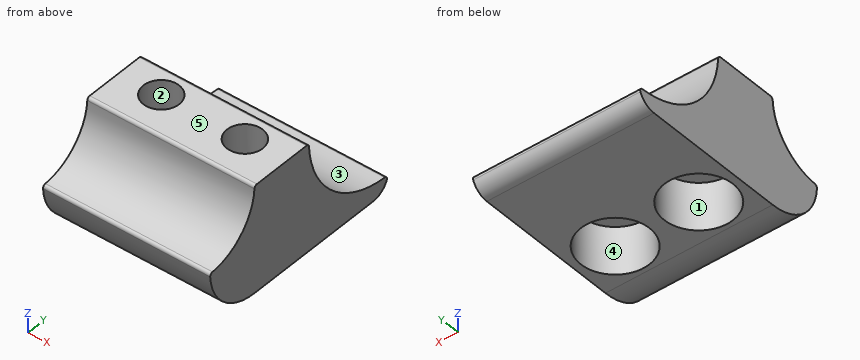
Autodesk Inventor part; units mm, degrees
ref_plane "YZ Plane" through (0, 0, 0) normal (1, 0, 0) x (0, 1, 0)
ref_plane "XZ Plane" through (0, 0, 0) normal (0, 1, 0) x (-1, 0, 0)
ref_plane "XY Plane" through (0, 0, 0) normal (0, 0, 1) x (1, 0, 0)
sketch "Szkic1" plane through (0, 0, 0) normal (0, 0, 1) x (1, 0, 0)
  line L0 (-14, 18) -> (14, 18)
  line L1 (14, 18) -> (14, -18)
  line L2 (14, -18) -> (-14, -18)
  line L3 (-14, -18) -> (-14, 18)
  line L4 (-14, 18) -> (14, -18) construction
  line L5 (14, 18) -> (-14, -18) construction
  point P0 (0, 0)
  dimension "d0" = 28
  dimension "d1" = 36
extrude "Wyciągnięcie proste1" add sketch "Szkic1" along normal mid plane 18
sketch "Szkic3" plane through (0, 0, 0) normal (1, 0, 0) x (0, 1, 0)
  line L0 (-18, 9) -> (-18, -9) construction
  line L1 (-18, 9) -> (18, 9) construction
  line L2 (18, 9) -> (18, -9) construction
  circle A0 centre (-18, 9) radius 9
  circle A1 centre (18, 9.5) radius 16
  point P0 (0, 0)
  dimension "d4" = 18
  dimension "d6" = 32
  dimension "d7" = 0.5
extrude "Wyciągnięcie proste2" cut sketch "Szkic3" along normal mid plane 28
fillet "Zaokrąglenie1" radius 3 1 edges at (0, 18, -9)
fillet "Zaokrąglenie2" radius 9 1 edges at (0, -18, -9)
fillet "Zaokrąglenie3" radius 0.5 5 edges at (0, -9, 9) (0, 2.0078, 9) (0, -18, -0.0001) (0, -18, 0) (0, 18, -6.5)
sketch "Szkic4" plane through (0, 0, -9) normal (0, 0, -1) x (-1, 0, 0)
  line L0 (14, -9) -> (-14, -9)
  line L1 (14, -9) -> (14, 15.042)
  line L2 (-14, 15.042) -> (14, 15.042)
  line L3 (-14, 15.042) -> (-14, -9)
  line L4 (-14, 2.0294) -> (14, 2.0294)
  line L5 (14, -9.0125) -> (-14, -9.0125)
  line L6 (0, 0) -> (0, 3.9534) construction
  point P0 (-7, -2.4906)
  point P1 (7, -2.4906)
  point P2 (-12.5, 2.0294)
  point P3 (12.5, 2.0294)
  point P4 (12.5, -7.0104)
  point P5 (-12.5, -7.0104)
  dimension "d14" = 4.52
  dimension "d15" = 14
hole "Otwór1" at (7, -2.4906, -9) at (-7, -2.4906, -9) direction (0, 0, 1) diameter 6 end through all counterbore diameter 11.5 counterbore depth 8
properties part number "Zawias" material "Stal nierdzewna"
Design review of the part built by this model. Coordinates are the model's own, in mm. Face numbers are marked on the shaded views. A direction names the side the tool comes from. Round coordinates to 2 decimals unless told otherwise and drop trailing zeros. Write each loop counter-clockwise with the first axis right and the second up, starting at its lowest first coordinate (ties: lowest second). Pieces come first, ordered by that corner, then holes. Notation, with made-up numbers: M -5,71.25 L 51,71.25 A36 ccw 51,105.25 Z; hole C 60.5,84.25 d11. An arc over 180 degrees is marked long. One line per item, written item: value. Start each with the question number.
1. Draft analysis for pull direction Y (two halves, no side actions). For the marked faces 3, 4 and 5, state which applies: pulls with the +Y half, pulls with the -Y half, needs draft (parallel to the pull), parting line crosses it, or undercut.
2. Take a section at A-A on z = 1.5. State the section outline as (x, y) points.
3. Clearance check with flat-ended pins moving along their axes: P1, Ø9, axis at x = 6.5, y = -2.5, coming from the -Z side; P2, Ø4, axis at x = -6.5, y = 14, coming from the +Z side; P3, Ø2, axis at x = 7, z = 2, coming from the +Y side. State where each tip first meets the part, or that it passes through.
4. For the marked faces 1 and 2, list the 3-axis set-ups (+Z, -Z, +X, -X, +Y, -Y) from which the entire face can be reached by the end or side of a thin tool; tool diameter is ignored.
5. To check wall thickness, follow probe 1 along X at (y, z) = (-3, 4); probe 2 along X at (y, z) = (-7.5, -4.75); probe 3 along Y at (x, z) = (-7, -4). State the ranges of each line that lie inside material, in increasing order. Write a range as from..to.
6. Take a section at C-C on y = -15. State the section outline as (x, z) points, then the cut area to 3 significant figures.
7. Take a section at B-B on z = -3. State the section outline as (x, y) points, then the cut area to 3 significant figures.
8. Take a section at D-D on y = 7. State the section outline as (x, z) points.
Computed:
1. face 3: pulls with the +Y half
1. face 4: undercut
1. face 5: needs draft
2. outline: M -14,-13.03 L 14,-13.03 L 14,4.14 L -14,4.14 Z; hole C -7,-2.49 d6; hole C 7,-2.49 d6
3. P1: stops at z = -1
3. P2: stops at z = -5.33
3. P3: stops at y = 4.44
4. face 1: -Z
4. face 2: +Z, -Z
5. probe 1: x = -14..-9.96, -4.04..4.04, 9.96..14
5. probe 2: x = -14..-9.82, -4.18..4.18, 9.82..14
5. probe 3: y = -17.06..-8.24, 3.26..9.41
6. outline: M -14,-6.71 L 14,-6.71 L 14,0.51 L -14,0.51 Z
6. area: 202 mm²
7. outline: M -14,-17.49 L 14,-17.49 L 14,8.01 L -14,8.01 Z; hole C -7,-2.49 d11.5; hole C 7,-2.49 d11.5
7. area: 506 mm²
8. outline: M -14,-9 L 14,-9 L 14,-2.12 L -14,-2.12 Z
